Can you work these out from the model? Positions are in its coordinate system, mm. A direction names the side the tool comes from. Give positions to 0.01 mm unless a question says otherwise; leave off trailing zeros. Write each loop counter-clockwise with the first axis right and the second up, starting at its lowest first coordinate (ties: lowest second). Pieces come first, ordered by that corner, then holes.
from build123d import *
from build123d.topology import SkipClean

# Parameters (mm, degrees)
SKETCH1_W           = 38
SKETCH1_H           = 40
BOSS_EXTRUDE1_DEPTH = 8
SKETCH2_R           = 7.5
SKETCH2_R_2         = 3.175
BOSS_EXTRUDE2_DEPTH = 5
FILLET1_R           = 1
CUT_EXTRUDE1_DEPTH  = 5.55625
SKETCH4_R           = 3.175
CUT_EXTRUDE2_DEPTH  = 57.683330883


with BuildPart() as part:
    # Sketch1 → Boss-Extrude1 (new body)
    with BuildSketch(Plane.XY):
        with Locations((19, 20)):
            Rectangle(SKETCH1_W, SKETCH1_H)
    extrude(amount=BOSS_EXTRUDE1_DEPTH)

    # Sketch2 → Boss-Extrude2 (add)
    with BuildSketch(Plane.XY.offset(8)):
        with Locations((19, 20)):
            Circle(SKETCH2_R)
        with Locations((19, 20)):
            Circle(SKETCH2_R_2, mode=Mode.SUBTRACT)
    extrude(amount=BOSS_EXTRUDE2_DEPTH)

    # Fillet1
    fillet1_edges = [part.edges().sort_by_distance(p)[0] for p in [
        (38, 20, 8),
        (11.5, 20, 8),
        (11.5, 20, 13),
        (19, 40, 8),
        (0, 20, 8),
        (19, 40, 0),
        (38, 20, 0),
        (19, 0, 0),
        (0, 20, 0),
        (0, 40, 4),
        (38, 40, 4),
        (38, 0, 4),
        (0, 0, 4),
        (19, 0, 8),
    ]]
    fillet(fillet1_edges, radius=FILLET1_R)

    # Sketch3 → Cut-Extrude1 (cut)
    with BuildSketch(Plane(origin=(0, 0, 0), x_dir=(-1, 0, 0), z_dir=(0, 0, -1))):
        Polygon((-15.791953229, 25.5565), (-22.208046771, 25.5565), (-25.416093542, 20), (-22.208046771, 14.4435), (-15.791953229, 14.4435), (-12.583906458, 20), align=None)
    extrude(amount=-CUT_EXTRUDE1_DEPTH, mode=Mode.SUBTRACT)

    # Sketch4 → Cut-Extrude2 (cut, through all)
    with SkipClean():  # the faces are left unmerged after this step: merging them gives an invalid solid
        with BuildSketch(Plane(origin=(0, 0, 0), x_dir=(-1, 0, 0), z_dir=(0, 0, -1))):
            with Locations((-19, 20)):
                Circle(SKETCH4_R)
        extrude(amount=-CUT_EXTRUDE2_DEPTH, mode=Mode.SUBTRACT)


solid = part.part
(1) If we mould it in two halves opening along Y, with no side actions, what happens to faces 1 (the face through (19, 0, 4)), 2 (the face through (13.5, 25.1, 10.5)), 3 (the face through (22.17, 20.14, 9.23)), 4 (the face through (0.285, 39.699, 4.042))? For each: +Y half, -Y half, draft (parallel to the pull), parting line (faces both ways), or undercut.
Returned:
face 1: -Y half
face 2: parting line
face 3: undercut
face 4: +Y half
(2) Imagine slicing it at C-C, the plane x = 31. Write out the boundary of the cut face in (y, z), plus the area to 3 significant figures.
Returned:
outline: (0, 1) arc R1 ccw to (1, 0) - (39, 0) arc R1 ccw to (40, 1) - (40, 7) arc R1 ccw to (39, 8) - (1, 8) arc R1 ccw to (0, 7) - close
area: 319 mm2
(3) For faces 5 (the face through (0.285, 0.301, 4.042)), 6 (the face through (19, 29, 8)), 7 (the face through (23.8, 22.8, 2.7)), which set-ups out of +Z, -Z, +X, -X, +Y, -Y let a thin tool reach every point of the face, with its end or its side?
Returned:
face 5: +Z, -Z, -X, -Y
face 6: +Z
face 7: -Z
(4) Imagine slicing it at A-A, the plane x = 19. Write out the boundary of the cut face in (y, z) (1 decimal).
Returned:
outline: (0, 1) arc R1 ccw to (1, 0) - (14.4, 0) - (14.4, 5.6) - (16.8, 5.6) - (16.8, 13) - (13.5, 13) arc R1 ccw to (12.5, 12) - (12.5, 9) arc R1 cw to (11.5, 8) - (1, 8) arc R1 ccw to (0, 7) - close; (23.2, 5.6) - (25.6, 5.6) - (25.6, 0) - (39, 0) arc R1 ccw to (40, 1) - (40, 7) arc R1 ccw to (39, 8) - (28.5, 8) arc R1 cw to (27.5, 9) - (27.5, 12) arc R1 ccw to (26.5, 13) - (23.2, 13) - close
(5) Imagine slicing it at B-B, the plane z = 2.5. Write out the boundary of the cut face in (x, y).
Returned:
outline: (0, 1) arc R1 ccw to (1, 0) - (37, 0) arc R1 ccw to (38, 1) - (38, 39) arc R1 ccw to (37, 40) - (1, 40) arc R1 ccw to (0, 39) - close; hole (12.58, 20) - (15.79, 14.44) - (22.21, 14.44) - (25.42, 20) - (22.21, 25.56) - (15.79, 25.56) - close
(6) If I drill on L1, parallel to Y at x = 19, z = 9.75 (3 decimals); L2, parallel to Y at x = 17, z = 1.75; L3, parallel to Z at x = 25.5, y = 31.5, over which ranges is the centre line in solid material (lowest first)?
Returned:
L1: y = 12.5 to 16.825, 23.175 to 27.5
L2: y = 0 to 14.44, 25.56 to 40
L3: z = 0 to 8
(7) Imagine slicing it at D-D, the plane y = 33. Write out the boundary of the cut face in (x, z), plus the area to 3 significant figures.
Returned:
outline: (0, 1) arc R1 ccw to (1, 0) - (37, 0) arc R1 ccw to (38, 1) - (38, 7) arc R1 ccw to (37, 8) - (1, 8) arc R1 ccw to (0, 7) - close
area: 303 mm2
